```python
from build123d import *

# Parameters (mm, degrees)
SKETCH1_W           = 38
SKETCH1_H           = 7
BOSS_EXTRUDE1_DEPTH = 2
SKETCH2_W           = 6.498713404
SKETCH2_H           = 7
SKETCH2_W_2         = 6.49777259
BOSS_EXTRUDE2_DEPTH = 1
SKETCH3_R           = 1
CUT_EXTRUDE1_DEPTH  = 3


with BuildPart() as part:
    # Sketch1 → Boss-Extrude1 (new body)
    with BuildSketch(Plane(origin=(0, 0, 0), x_dir=(1, 0, 0), z_dir=(0, 1, 0))):
        Rectangle(SKETCH1_W, SKETCH1_H)
    extrude(amount=BOSS_EXTRUDE1_DEPTH)

    # Sketch2 → Boss-Extrude2 (add)
    with BuildSketch(Plane(origin=(0, 2, 0), x_dir=(1, 0, 0), z_dir=(0, 1, 0))):
        with Locations((-15.750643298, 0)):
            Rectangle(SKETCH2_W, SKETCH2_H)
        with Locations((15.751113705, 0)):
            Rectangle(SKETCH2_W_2, SKETCH2_H)
    extrude(amount=BOSS_EXTRUDE2_DEPTH)

    # Sketch3 → Cut-Extrude1 (cut)
    with BuildSketch(Plane(origin=(0, 3, 0), x_dir=(1, 0, 0), z_dir=(0, 1, 0))):
        with Locations(Location((-16.001286596, 0, 0), (0, 0, 270))):
            Circle(SKETCH3_R)
        with Locations(Location((16.00222741, 0, 0), (0, 0, 270))):
            Circle(SKETCH3_R)
    extrude(amount=-CUT_EXTRUDE1_DEPTH, mode=Mode.SUBTRACT)


solid = part.part
```
Model file for the job. Use its own axes, mm. A direction names the side the tool comes from. Give positions to 0.01 mm unless a question says otherwise; leave off trailing zeros. Write each loop counter-clockwise with the first axis right and the second up, starting at its lowest first coordinate (ties: lowest second). Pieces come first, ordered by that corner, then holes. Notation, with made-up numbers: (35.5, -36.5) -> (58.5, -36.5) arc R25 cw to (58.5, -7.5) -> close; hole circle Ø10 at (1.5, 70). An arc over 180 degrees is marked (long way). Use CSV: the item, a comma, the result in double quotes. Start each with the question number.
1) Cut at D-D on x = 6. List the corners of the cut face in (y, z).
2) Drill centre lines: L1, parallel to X at y = 0.9, z = 0; L2, parallel to X at y = 2.6, z = 2.5; L3, parallel to X at y = 2.9, z = 0.75. Where is each one in solid material? Low to high.
3) Two-plate mould, pull along X, no slides. Class faces 1 (the cylindrical face through (-17, 2, 0)), 2 (the flat face through (-19, 1, 0)), 3 (the flat face through (0, 2, 0)), 4 (the flat face through (15, 3, -1)): released by +X, released by -X, zero draft, split by the parting line, or undercut.
4) Tool access for faces 5 (the flat face through (-15, 3, -1)), 6 (the flat face through (-12.501, 2.5, 0)): list every direction of +Z, -Z, +X, -X, +Y, -Y with a clear straight run to the whole face (end or side of a thin tool).
5) Cut at B-B on y = 2.6. List the corners of the cut face in (x, z).
6) Cut at A-A on z = 0. List the corners of the cut face in (x, y).
7) Pin check, flat tips, straight feed: P1, Ø2, axis at x = 10.5, z = -1.5, coming from the +Y side; P2, Ø1.6, axis at x = 16, z = 0, coming from the -Y side. Stop position of each tip, or through.
8) Cut at C-C on z = 2.5. List the corners of the cut face in (x, y), plus the area to 3 significant figures.
Final values:
1,outline,"(0, -3.5) -> (2, -3.5) -> (2, 3.5) -> (0, 3.5) -> close"
2,L1,"x = -19 to -17, -15 to 15, 17 to 19"
2,L2,"x = -19 to -12.5, 12.5 to 19"
2,L3,"x = -19 to -16.66, -15.34 to -12.5, 12.5 to 15.34, 16.66 to 19"
3,face 1,"undercut"
3,face 2,"released by -X"
3,face 3,"undercut"
3,face 4,"zero draft"
4,face 5,"+Z, -Z, +X, -X, +Y"
4,face 6,"+Z, -Z, +Y"
5,outline,"(-19, -3.5) -> (-12.5, -3.5) -> (-12.5, 3.5) -> (-19, 3.5) -> close; (12.5, -3.5) -> (19, -3.5) -> (19, 3.5) -> (12.5, 3.5) -> close; hole circle Ø2 at (-16, 0); hole circle Ø2 at (16, 0)"
6,outline,"(-19, 0) -> (-17, 0) -> (-17, 3) -> (-19, 3) -> close; (-15, 0) -> (15, 0) -> (15, 3) -> (12.5, 3) -> (12.5, 2) -> (-12.5, 2) -> (-12.5, 3) -> (-15, 3) -> close; (17, 0) -> (19, 0) -> (19, 3) -> (17, 3) -> close"
7,P1,"stops at y = 2"
7,P2,"passes through"
8,outline,"(-19, 0) -> (19, 0) -> (19, 3) -> (12.5, 3) -> (12.5, 2) -> (-12.5, 2) -> (-12.5, 3) -> (-19, 3) -> close"
8,area,"89.0 mm2"
